Work out the finished part from the listing and answer in its coordinate system (mm). Face numbers are marked on the shaded views. Give positions to 0.01 mm unless a question says otherwise; leave off trailing zeros. Order: outer loops, then holes, each group sorted by start corner. A loop starts at its lowest first (then second) coordinate and runs counter-clockwise, first axis right, second up.
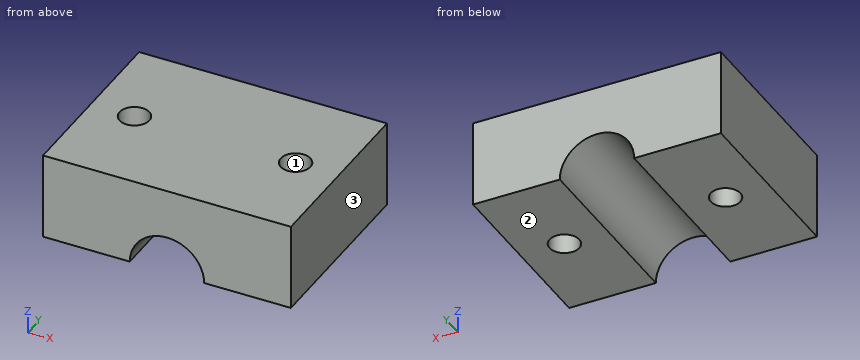
```python
from build123d import *

# Parameters (mm, degrees)
SKETCH1_W          = 20
SKETCH1_H          = 15
EXTRUDE1_DEPTH     = 3.5
SKETCH2_R          = 3
CUT_EXTRUDE1_DEPTH = 16
SKETCH3_R          = 1.2
CUT_EXTRUDE2_DEPTH = 8


with BuildPart() as part:
    # Sketch1 → Extrude1 (new body, symmetric)
    with BuildSketch(Plane.XY):
        Rectangle(SKETCH1_W, SKETCH1_H)
    extrude(amount=EXTRUDE1_DEPTH, both=True)

    # Sketch2 → Cut-Extrude1 (cut, through all)
    with BuildSketch(Plane(origin=(0, 7.5, 0), x_dir=(-1, 0, 0), z_dir=(0, 1, 0))):
        with Locations((0, -3.5)):
            Circle(SKETCH2_R)
    extrude(amount=-CUT_EXTRUDE1_DEPTH, mode=Mode.SUBTRACT)

    # Sketch3 → Cut-Extrude2 (cut, through all)
    with BuildSketch(Plane.XY.offset(3.5)):
        with Locations((-6.5, 0)):
            Circle(SKETCH3_R)
        with Locations((6.5, 0)):
            Circle(SKETCH3_R)
    extrude(amount=-CUT_EXTRUDE2_DEPTH, mode=Mode.SUBTRACT)


solid = part.part
```
1. The mould has two halves that part along X. Classify the marked faces 1, 2 and 3: pulls with the +X half, pulls with the -X half, needs draft (parallel to the pull), parting line crosses it, or undercut.
Findings below:
face 1: undercut
face 2: needs draft
face 3: pulls with the +X half
2. Straight lines are drawn through the part: probe 1 along Y at (x, z) = (-6.5, 2); probe 2 along X at (y, z) = (0.5, 0); probe 3 along Y at (x, z) = (7, -2.5). For each, find the intervals that lie inside material, in ascending order.
Findings below:
probe 1: y = -7.5 to -1.2, 1.2 to 7.5
probe 2: x = -10 to -7.59, -5.41 to 5.41, 7.59 to 10
probe 3: y = -7.5 to -1.09, 1.09 to 7.5
3. The part is cut by section D-D (z = 2). Write down the section's boundary in (x, y).
Findings below:
outline: (-10, -7.5) - (10, -7.5) - (10, 7.5) - (-10, 7.5) - close; hole circle Ø2.4 at (-6.5, 0); hole circle Ø2.4 at (6.5, 0)
4. The part is cut by section A-A (y = 0). Write down the section's boundary in (x, z), then the cut area to 3 significant figures.
Findings below:
outline: (-10, -3.5) - (-7.7, -3.5) - (-7.7, 3.5) - (-10, 3.5) - close; (-5.3, -3.5) - (-3, -3.5) arc R3 cw to (3, -3.5) - (5.3, -3.5) - (5.3, 3.5) - (-5.3, 3.5) - close; (7.7, -3.5) - (10, -3.5) - (10, 3.5) - (7.7, 3.5) - close
area: 92.3 mm2
5. The part is cut by section C-C (x = 6.5). Write down the section's boundary in (y, z).
Findings below:
outline: (-7.5, -3.5) - (-1.2, -3.5) - (-1.2, 3.5) - (-7.5, 3.5) - close; (1.2, -3.5) - (7.5, -3.5) - (7.5, 3.5) - (1.2, 3.5) - close
6. Given P1, Ø4, axis at x = -6.5, y = 0, coming from the -Z side, flat-ended and moving along its own axis, determine where the tip first touches the part or whether it passes through.
Findings below:
P1: stops at z = -3.5
7. The part is cut by section B-B (z = -2.5). Write down the section's boundary in (x, y), then the cut area to 3 significant figures.
Findings below:
outline: (-10, -7.5) - (-2.83, -7.5) - (-2.83, 7.5) - (-10, 7.5) - close; (2.83, -7.5) - (10, -7.5) - (10, 7.5) - (2.83, 7.5) - close; hole circle Ø2.4 at (-6.5, 0); hole circle Ø2.4 at (6.5, 0)
area: 206 mm2
